Autodesk Inventor part; units mm, degrees
ref_plane "YZ Plane" through (0, 0, 0) normal (1, 0, 0) x (0, 1, 0)
ref_plane "XZ Plane" through (0, 0, 0) normal (0, 1, 0) x (-1, 0, 0)
ref_plane "XY Plane" through (0, 0, 0) normal (0, 0, 1) x (1, 0, 0)
sketch "スケッチ2" plane through (0, 0, 0) normal (0, 1, 0) x (-1, 0, 0)
  arc A0 (186.0286, -63.1802) -> (352.6649, -47.4935) centre (165.9229, 1043.3137) ccw
  arc A1 (138.8299, -62.6406) -> (186.0286, -63.1802) centre (171.5405, 734.1521) ccw
  arc A2 (52.1426, -47.2314) -> (138.8299, -62.6406) centre (152.2575, 264.4411) ccw
  arc A3 (2.1008, -22.6524) -> (52.1426, -47.2314) centre (110.8425, 135.5101) ccw
  arc A4 (-12.1054, -8.8578) -> (2.1008, -22.6524) centre (35.5695, 26.0271) ccw
  arc A5 (-4.5779, 14.2844) -> (-12.1054, -8.8578) centre (0, 0) ccw
  arc A6 (16.7232, 17.0724) -> (-4.5779, 14.2844) centre (13.7336, -42.8531) ccw
  arc A7 (94.7165, 2.6851) -> (16.7232, 17.0724) centre (1.7751, -282.555) ccw
  arc A8 (94.7165, 2.6851) -> (99.4705, 1.147) centre (466.4821, 1143.6454) ccw
  arc A9 (99.4705, 1.147) -> (352.0248, -39.551) centre (359.437, 810.4167) ccw
  arc A10 (352.6649, -47.4935) -> (352.0248, -39.551) centre (351.99, -43.5508) ccw
  circle A11 centre (33.0346, -3.4541) radius 6
  circle A12 centre (243.4846, -47.452) radius 6
  point P0 (0, 0)
extrude "押し出し2" add sketch "スケッチ2" along normal mid plane 186
ref_plane "作業平面1" through (-10.8988, -64, -64.8158) normal (0.2588, 0, -0.9659) x (0, -1, 0)
ref_plane "作業平面2" through (-226.5252, -64, -89.4952) normal (-0.2588, 0, 0.9659) x (-0.9659, 0, -0.2588)
sketch "スケッチ3" plane through (-10.8988, -64, -64.8158) normal (0.2588, 0, -0.9659) x (0, -1, 0)
  line L0 (25, -7) -> (0, -7)
  line L1 (0, -7) -> (0, 18)
  line L2 (0, 18) -> (25, 18)
  line L3 (25, 18) -> (25, -7)
  line L4 (-1, -8) -> (26, -8)
  line L5 (26, -8) -> (26, 19)
  line L6 (26, 19) -> (-1, 19)
  line L7 (-1, 19) -> (-1, -8)
  point P0 (-64, -27.303)
  dimension "d6" = 1
extrude "押し出し3" cut sketch "スケッチ3" against normal blind 75 contours L0 L1 L2 L3 | L7 L6 L5 L4
sketch "スケッチ4" plane through (-226.5252, -64, -89.4952) normal (-0.2588, 0, 0.9659) x (-0.9659, 0, -0.2588)
  line L0 (-7, 25) -> (-7, 0)
  line L1 (-7, 0) -> (18, 0)
  line L2 (18, 0) -> (18, 25)
  line L3 (18, 25) -> (-7, 25)
  line L4 (-8, -1) -> (-8, 26)
  line L5 (-8, 26) -> (19, 26)
  line L6 (19, 26) -> (19, -1)
  line L7 (19, -1) -> (-8, -1)
  point P0 (-241.9696, -64)
  dimension "d9" = 1
extrude "押し出し4" cut sketch "スケッチ4" along normal blind 55 contours L3 L2 L1 L0 | L4 L5 L6 L7
properties part number "mainflap for side"
Read the model definition and answer for the solid it produces. Units are mm, in the model's axes. A direction names the side the tool comes from. Give positions to 0.01 mm unless a question says otherwise; leave off trailing zeros. Order: outer loops, then holes, each group sorted by start corner. A loop starts at its lowest first (then second) coordinate and runs counter-clockwise, first axis right, second up. Notation, with made-up numbers: (66.25, -20) -> (113.25, -20) arc R13 cw to (113.25, 4) -> close; hole circle Ø9 at (19.5, -19). An arc over 180 degrees is marked (long way). One line per item, written item: value. Start each with the question number.
(1) The part is cut by section C-C (x = -242). Determine the outline of the cut face in (y, z), and give its area (3 significant figures).
(2) A tool of negligible diameter and unlimited length cuts with its end or side. For faces 5 (the flat face through (-245.89, -76.69, -37.74)), 6 (the flat face through (-17.308, -76.311, -9.985)), 7 (the cylindrical face through (-355.97, -1.3, -43.15)), from which of +Z, -Z, +X, -X, +Y, -Y can it reach the whole face along a straight path? Write none if from no direction.
(3) The part is cut by section A-A (y = 34). Determine the outline of the cut face in (x, z), and give its area (3 significant figures).
(4) Straight lines are drawn through the part: L1, parallel to Z at x = -179, y = -27.5; L2, parallel to Z at x = -89.5, y = 8; L3, parallel to X at y = 14.5, z = -41. For each, find the intervals that lie inside material, in ascending order.
(5) The part is cut by section D-D (x = -81). Determine the outline of the cut face in (y, z).
(6) For a pull along Y with two mould halves and no side action, classify faces 1 (the cylindrical face through (-242.7, -91.5, -53.4)), 2 (the flat face through (-241, -90, -55)), 3 (the flat face through (-127, -93, -31)), 4 (the flat face through (-256.592, -76.689, -50.693)) as released by +Y, released by -Y, zero draft, split by the parting line, or undercut.
(7) Flat-ended cylindrical pins translate along their axes: P1, Ø9.5, axis at x = -33.03, z = -3.45, coming from the +Y side; P2, Ø1, axis at x = -71.5, y = -5.5, coming from the -Z side; P3, Ø3, axis at y = 35.5, z = -26, coming from the +X side; P4, Ø8, axis at y = 9, z = 8, coming from the +X side. Find the tip coordinate at first contact, or state that the pin passes through.
(8) The part is cut by section B-B (z = -14). Determine the outline of the cut face in (x, y).
Taken from the geometry:
1. outline: (-93, -60.74) -> (-90, -60.74) -> (-90, -53.27) -> (-93, -53.27) -> close; (-93, -41.64) -> (-90, -41.64) -> (-90, -36.7) -> (-63, -36.7) -> (-63, -41.64) -> (93, -41.64) -> (93, -31.43) -> (-93, -31.43) -> close; (-63, -60.74) -> (93, -60.74) -> (93, -53.27) -> (-63, -53.27) -> close
1. area: 2,950 mm^2
2. face 5: none
2. face 6: -Z
2. face 7: -X, +Y, -Y
3. outline: (-352.66, -47.49) arc R1106.67 ccw to (-186.03, -63.18) arc R797.54 ccw to (-138.83, -62.64) arc R327.36 ccw to (-52.14, -47.23) arc R191.94 ccw to (-2.1, -22.65) arc R59.07 ccw to (12.11, -8.86) arc R15 ccw to (4.58, 14.28) arc R60 ccw to (-16.72, 17.07) arc R300 ccw to (-94.72, 2.69) arc R1203.96 cw to (-99.47, 1.15) arc R850 cw to (-352.02, -39.55) arc R4 ccw to start; hole circle Ø12 at (-243.48, -47.45); hole circle Ø12 at (-33.03, -3.45)
3. area: 14,200 mm^2
4. L1: -63.28 to -20.21
4. L2: -56.84 to 4.33
4. L3: -355.07 to -35.45
5. outline: (-93, -55.07) -> (93, -55.07) -> (93, 6.8) -> (-93, 6.8) -> close
6. face 1: zero draft
6. face 2: undercut
6. face 3: released by -Y
6. face 4: undercut
7. P1: through
7. P2: z = -52.93
7. P3: x = -4.84
7. P4: x = 14.46
8. outline: (-152.47, -93) -> (7.88, -93) -> (7.88, 93) -> (-152.47, 93) -> close; hole (-44.19, -90) -> (-16.23, -90) -> (-16.23, -63) -> (-44.19, -63) -> close
